Part model, mm, in its own coordinate system. Face numbers are marked on the shaded views. Give positions to 0.01 mm unless a question says otherwise; leave off trailing zeros. Write each loop counter-clockwise with the first axis right and the second up, starting at its lowest first coordinate (ties: lowest second). Pieces come first, ordered by that corner, then holes. Notation, with made-up numbers: (70, 59) - (95, 59) arc R16 cw to (95, 67) - close; hole circle Ø4 at (48, 36.5). An arc over 180 degrees is marked (long way). Answer as a JSON object with one key per item and string values. Group by question number.
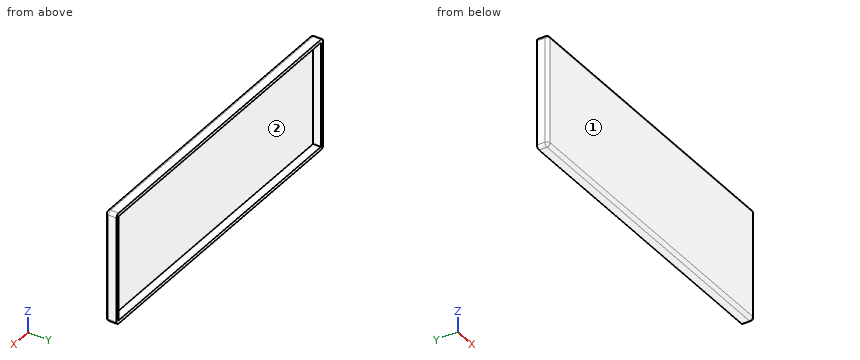
```python
from build123d import *

# Parameters (mm, degrees)
RECTANGLEBOX_DEPTH      = 5
RECTANGLEBOX_DEPTH_BACK = 2
SKETCHREC_W             = 200
SKETCHREC_H             = 70
RECTANGLER_R            = 2
RECTANGLEC_START        = -98
RECTANGLEC_OUTLINE_W    = 5
RECTANGLEC_OUTLINE_H    = 66
RECTANGLEC_DEPTH        = 196


# Read off the part's stored shape, not the designer's step: RectangleC
with BuildPart() as part:
    # SketchRec → RectangleBox (new, two sides: drawn at the far end of the back side and taken through both)
    with BuildSketch(Plane(origin=(0, 0, 0), x_dir=(1, 0, 0), z_dir=(0, 1, 0)).offset(-RECTANGLEBOX_DEPTH_BACK)):
        Rectangle(SKETCHREC_W, SKETCHREC_H)
    extrude(amount=RECTANGLEBOX_DEPTH + RECTANGLEBOX_DEPTH_BACK)

    # RectangleR
    rectangler_edges = [part.edges().sort_by_distance(p)[0] for p in [
        (-100, -2, 0),
        (0, -2, 35),
        (100, -2, 0),
        (0, -2, -35),
        (100, 1.5, 35),
        (-100, 1.5, 35),
        (-100, 1.5, -35),
        (100, 1.5, -35),
    ]]
    fillet(rectangler_edges, radius=RECTANGLER_R)

    # RectangleC outline → RectangleC (cut)
    with BuildSketch(Plane.YZ.offset(RECTANGLEC_START)):
        with Locations((2.5, 0)):
            Rectangle(RECTANGLEC_OUTLINE_W, RECTANGLEC_OUTLINE_H)
    extrude(amount=RECTANGLEC_DEPTH, mode=Mode.SUBTRACT)


solid = part.part
```
1) Band-saw the part on C-C (z = -8). List the corners of the cut face in (x, y), plus the area to 3 significant figures.
2) Band-saw the part on B-B (x = 18). List the corners of the cut face in (y, z), plus the area to 3 significant figures.
3) Drop a flat-ended pin along its axis: P1, Ø1.5, axis at x = 33.5, z = 8.5, coming from the +Y side. Give the stop position or say it passes through.
4) Band-saw the part on A-A (y = 3.5). List the corners of the cut face in (x, z), plus the area to 3 significant figures.
5) Probe line 1 (Z direction, x = -72, y = 4); line 2 (X direction, y = 3.75, z = 13.5); line 3 (Z direction, x = 8, y = -0.25). List the from-to ranges inside material, lowest first.
6) Mould opens along Z. For the marked faces 1 and 2 say: pulls with the +Z half, pulls with the -Z half, needs draft (parallel to the pull), parting line crosses it, or undercut.
Verdict:
{
 "1": {"outline": "(-100, 0) arc R2 ccw to (-98, -2) - (98, -2) arc R2 ccw to (100, 0) - (100, 5) - (98, 5) - (98, 0) - (-98, 0) - (-98, 5) - (-100, 5) - close", "area": "418 mm2"},
 "2": {"outline": "(-2, -33) arc R2 ccw to (0, -35) - (5, -35) - (5, -33) - (0, -33) - (0, 33) - (5, 33) - (5, 35) - (0, 35) arc R2 ccw to (-2, 33) - close", "area": "158 mm2"},
 "3": {"P1": "y = 0"},
 "4": {"outline": "(-100, -33) arc R2 ccw to (-98, -35) - (98, -35) arc R2 ccw to (100, -33) - (100, 33) arc R2 ccw to (98, 35) - (-98, 35) arc R2 ccw to (-100, 33) - close; hole (-98, -33) - (98, -33) - (98, 33) - (-98, 33) - close", "area": "1,060 mm2"},
 "5": {"line 1": "-35 to -33, 33 to 35", "line 2": "-100 to -98, 98 to 100", "line 3": "-34.98 to 34.98"},
 "6": {"face 1": "needs draft", "face 2": "undercut"}
}
